Could you check a few things on this model? Use its own coordinates, in mm. A direction names the side the tool comes from. Coordinates: 2 decimals unless noted, no trailing zeros. Loops run counter-clockwise (first coordinate to the right, second up) from the corner with the lowest first, then second, coordinate; pieces in that order, holes last. Notation, with made-up numbers: (81.25, 82) - (114.25, 82) arc R26 ccw to (114.25, 106) - close; hole circle Ø5 at (84.5, -5). An arc over 180 degrees is marked (long way). Use CSV: the item, a comma, the result in double quotes.
from build123d import *

# Parameters (mm, degrees)
SKETCH1_W           = 155
SKETCH1_H           = 110
BOSS_EXTRUDE1_DEPTH = 4
SKETCH2_W           = 55
SKETCH2_H           = 35
SKETCH2_R           = 1.5
CUT_EXTRUDE1_DEPTH  = 148
FILLET2_R           = 15
FILLET3_R           = 7
SKETCH3_W           = 45
SKETCH3_H           = 26.5
BOSS_EXTRUDE2_DEPTH = 3
SKETCH5_W           = 45
SKETCH5_H           = 5
BOSS_EXTRUDE3_DEPTH = 33
SKETCH6_R           = 4
SKETCH6_R_2         = 1.5
CUT_EXTRUDE2_DEPTH  = 223
FILLET4_R           = 10
FILLET5_R           = 1
SKETCH9_W           = 119.31184044
SKETCH9_H           = 34
CUT_EXTRUDE4_DEPTH  = 1
FILLET8_R           = 4
SKETCH10_W          = 5
SKETCH10_H          = 3
CUT_EXTRUDE5_DEPTH  = 4


with BuildPart() as part:
    # Sketch1 → Boss-Extrude1 (new body)
    with BuildSketch(Plane.XY):
        Rectangle(SKETCH1_W, SKETCH1_H)
    extrude(amount=BOSS_EXTRUDE1_DEPTH)

    # Sketch2 → Cut-Extrude1 (cut)
    with BuildSketch(Plane.XY.offset(4)):
        with Locations((50, -37.5)):
            Rectangle(SKETCH2_W, SKETCH2_H)
        with Locations((50, 37.5)):
            Rectangle(SKETCH2_W, SKETCH2_H)
        with Locations((-71.5, 49)):
            Circle(SKETCH2_R)
        with Locations(Location((-71.5, -49, 0), (0, 0, 180))):
            Circle(SKETCH2_R)
        with Locations((71, 13.5)):
            Circle(SKETCH2_R)
        with Locations(Location((71, -13.5, 0), (0, 0, 180))):
            Circle(SKETCH2_R)
        with Locations((13.5, 49)):
            Circle(SKETCH2_R)
        with Locations(Location((13.5, -49, 0), (0, 0, 180))):
            Circle(SKETCH2_R)
    extrude(amount=-CUT_EXTRUDE1_DEPTH, mode=Mode.SUBTRACT)

    # Fillet2
    fillet2_edges = [part.edges().sort_by_distance(p)[0] for p in [
        (22.5, 20, 2),
        (22.5, -20, 2),
    ]]
    fillet(fillet2_edges, radius=FILLET2_R)

    # Fillet3
    fillet3_edges = [part.edges().sort_by_distance(p)[0] for p in [
        (77.5, 20, 2),
        (77.5, -20, 2),
    ]]
    fillet(fillet3_edges, radius=FILLET3_R)

    # Sketch3 → Boss-Extrude2 (add)
    with BuildSketch(Plane.XY.offset(4)):
        with Locations((-35, 68.25)):
            Rectangle(SKETCH3_W, SKETCH3_H)
        with Locations((-35, -68.25)):
            Rectangle(SKETCH3_W, SKETCH3_H)
    extrude(amount=-BOSS_EXTRUDE2_DEPTH)

    # Sketch5 → Boss-Extrude3 (add)
    with BuildSketch(Plane.XY.offset(4)):
        with Locations((-35, 79)):
            Rectangle(SKETCH5_W, SKETCH5_H)
        with Locations((-35, -79)):
            Rectangle(SKETCH5_W, SKETCH5_H)
    extrude(amount=BOSS_EXTRUDE3_DEPTH)

    # Sketch6 → Cut-Extrude2 (cut)
    with BuildSketch(Plane(origin=(0, 81.5, 0), x_dir=(1, 0, 0), z_dir=(0, 1, 0))):
        with Locations(Location((-35, -19.5, 0), (0, 0, 270))):
            Circle(SKETCH6_R)
        with Locations(Location((-43.5, -19.5, 0), (0, 0, 270))):
            Circle(SKETCH6_R_2)
        with Locations(Location((-26.5, -19.5, 0), (0, 0, 270))):
            Circle(SKETCH6_R_2)
    extrude(amount=-CUT_EXTRUDE2_DEPTH, mode=Mode.SUBTRACT)

    # Fillet4
    fillet4_edges = [part.edges().sort_by_distance(p)[0] for p in [
        (-12.5, 55, 2.5),
        (-57.5, 55, 2.5),
        (-57.5, -55, 2.5),
        (-12.5, -55, 2.5),
    ]]
    fillet(fillet4_edges, radius=FILLET4_R)

    # Fillet5
    fillet5_edges = [part.edges().sort_by_distance(p)[0] for p in [
        (-35, 76.5, 4),
        (-35, -76.5, 4),
    ]]
    fillet(fillet5_edges, radius=FILLET5_R)

    # Sketch9 → Cut-Extrude4 (cut)
    with BuildSketch(Plane.XY.offset(4)):
        with Locations((7.15592022, 0)):
            Rectangle(SKETCH9_W, SKETCH9_H)
    extrude(amount=-CUT_EXTRUDE4_DEPTH, mode=Mode.SUBTRACT)

    # Fillet8
    fillet8_edges = [part.edges().sort_by_distance(p)[0] for p in [
        (22.5, 55, 2),
        (22.5, -55, 2),
        (-77.5, 55, 2),
        (-77.5, -55, 2),
    ]]
    fillet(fillet8_edges, radius=FILLET8_R)

    # Sketch10 → Cut-Extrude5 (cut)
    with BuildSketch(Plane.XY.offset(4)):
        with Locations((-45, 23.5)):
            Rectangle(SKETCH10_W, SKETCH10_H)
        with Locations((-20, 23.5)):
            Rectangle(SKETCH10_W, SKETCH10_H)
        with Locations((10, 23.5)):
            Rectangle(SKETCH10_W, SKETCH10_H)
        with Locations((10, -23.5)):
            Rectangle(SKETCH10_W, SKETCH10_H)
        with Locations((-20, -23.5)):
            Rectangle(SKETCH10_W, SKETCH10_H)
        with Locations((-45, -23.5)):
            Rectangle(SKETCH10_W, SKETCH10_H)
    extrude(amount=-CUT_EXTRUDE5_DEPTH, mode=Mode.SUBTRACT)


solid = part.part
(1) Which directions (+Z, -Z, +X, -X, +Y, -Y) give clear straight access to the entire face, cutting with the end or side of a thin tool? Please do faces 5 (the face through (-18, 18, 4)), 6 (the face through (-12.5, 77, 15)), 7 (the face through (-20, 25, 2)), 8 (the face through (54, -20, 2)).
Computed:
face 5,"+Z, +X, -X"
face 6,"+Z, -Z, +X, +Y"
face 7,"+Z, -Z"
face 8,"+Z, -Z, +X, -Y"
(2) Please list where these lines run through material, in increasing order: line 1 (X direction, y = -49, z = 1.5); line 2 (Y direction, x = 13.5, z = 1.8); line 3 (Y direction, x = 71, z = 2).
Computed:
line 1,"x = -77.5 to -73, -70 to 12, 15 to 22.5"
line 2,"y = -55 to -50.5, -47.5 to 47.5, 50.5 to 55"
line 3,"y = -19.98 to -15, -12 to 12, 15 to 19.98"
(3) Suppose I cut it at B-B (x = -35). Write out the boundary of the cut face in (y, z), plus the area to 3 significant figures.
Computed:
outline,"(-81.5, 1) - (-55, 1) - (-55, 0) - (55, 0) - (55, 1) - (81.5, 1) - (81.5, 15.5) - (76.5, 15.5) - (76.5, 5) arc R1 cw to (75.5, 4) - (17, 4) - (17, 3) - (-17, 3) - (-17, 4) - (-75.5, 4) arc R1 cw to (-76.5, 5) - (-76.5, 15.5) - (-81.5, 15.5) - close; (-81.5, 23.5) - (-76.5, 23.5) - (-76.5, 37) - (-81.5, 37) - close; (76.5, 23.5) - (81.5, 23.5) - (81.5, 37) - (76.5, 37) - close"
area,"815 mm²"
(4) Thinking about a two-plate mould opening in X: for faces 1 (the face through (-45, 25, 2)), 2 (the face through (-35, 79, 37)), 3 (the face through (-57.5, -77, 15)), 4 (the face through (75.4, 18, 2)), which applies, +X half, -X half, draft (parallel to the pull), parting line (faces both ways), or undercut?
Computed:
face 1,"undercut"
face 2,"draft"
face 3,"-X half"
face 4,"+X half"
(5) Suppose I cut it at D-D (y = -58). Write out the boundary of the cut face in (x, z), plus the area to 3 significant figures.
Computed:
outline,"(-60.36, 1) - (-9.64, 1) - (-9.64, 4) - (-60.36, 4) - close"
area,"152 mm²"
(6) Will these pins go through, and if not, where does the flat tip stop? pin 1 (3 mm diameter, centred on x = -27, y = -13, fed in from -Z); pin 2 (8 mm diameter, centred on x = -24, y = 72, fed in from -Z); pin 3 (12 mm diameter, centred on y = 47.5, z = 9.5, fed in from +X); pin 4 (2.5 mm diameter, centred on x = 71, y = 13.5, fed in from -Z).
Computed:
pin 1,"stops at z = 0"
pin 2,"stops at z = 1"
pin 3,"stops at x = 22.5"
pin 4,"passes through"
(7) Suppose I cut it at A-A (z = 30). Write out the boundary of the cut face in (x, y), plus the area to 3 significant figures.
Computed:
outline,"(-57.5, -81.5) - (-12.5, -81.5) - (-12.5, -76.5) - (-57.5, -76.5) - close; (-57.5, 76.5) - (-12.5, 76.5) - (-12.5, 81.5) - (-57.5, 81.5) - close"
area,"450 mm²"
(8) Suppose I cut it at C-C (x = 4). Write out the boundary of the cut face in (y, z), plus the area to 3 significant figures.
Computed:
outline,"(-55, 0) - (55, 0) - (55, 4) - (17, 4) - (17, 3) - (-17, 3) - (-17, 4) - (-55, 4) - close"
area,"406 mm²"
